Can you work these out from the drawing? Everything is in mm from the part's minimum corner. Round coordinates to 2 decimals unless told otherwise and drop trailing zeros. Write each loop counter-clockwise with the first axis right and the second up, starting at its lowest first coordinate (ties: lowest second). Pieces come first, ordered by that corner, then holes. Notation, with made-up numbers: (-18.75, 35) - (20.25, 35) arc R26 cw to (20.25, 70) - close; hole circle Ø11 at (53, 4.25). An arc over 180 degrees is marked (long way). One line per item, written item: value. Start each with the question number.
Item 1: Imagine slicing it at A-A, the plane x = 19.5. Please give me the cut outline in (y, z).
Item 2: If I drill on line 1 (Y direction, x = 19.5, z = 0.85); line 2 (X direction, y = 3.25, z = 0.35); line 3 (Z direction, x = 15.5, y = 5.5), over which ranges is the centre line in solid material (lowest first)?
Item 3: For P1, Ø1.2, axis at y = 12.5, z = 2.5, coming from the -X side; P2, Ø1.5, axis at x = 3.5, y = 19.5, coming from the -Z side; P3, Ø3, axis at x = 19.5, y = 3.5, coming from the -Z side; P4, Ø1.6, axis at y = 12, z = 2.5, coming from the +X side, each with a flat end and sliding along its axis, tell me the tip position at first contact or that it passes through.
Item 4: Imagine slicing it at C-C, the plane z = 1.2. Please give me the cut outline in (x, y), then the cut area to 3 significant figures.
Item 5: Imagine slicing it at D-D, the plane x = 10.5. Please give me the cut outline in (y, z).
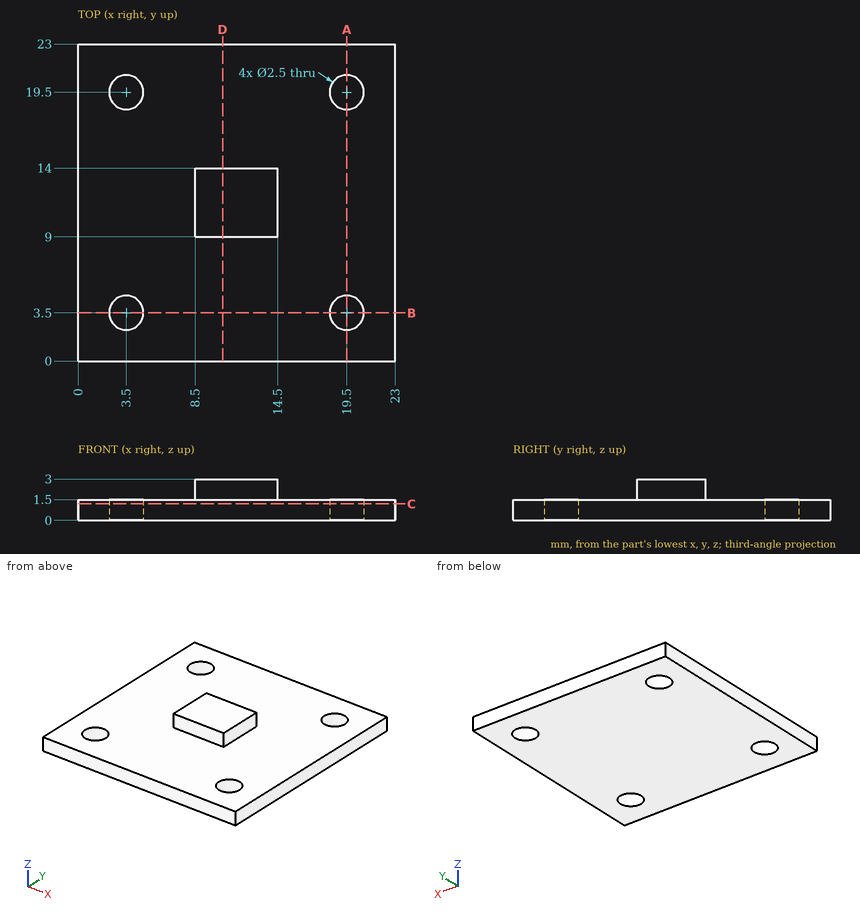
Values follow:
1. outline: (0, 0) - (2.25, 0) - (2.25, 1.5) - (0, 1.5) - close; (4.75, 0) - (18.25, 0) - (18.25, 1.5) - (4.75, 1.5) - close; (20.75, 0) - (23, 0) - (23, 1.5) - (20.75, 1.5) - close
2. line 1: y = 0 to 2.25, 4.75 to 18.25, 20.75 to 23
2. line 2: x = 0 to 2.28, 4.72 to 18.28, 20.72 to 23
2. line 3: z = 0 to 1.5
3. P1: stops at x = 8.5
3. P2: passes through
3. P3: stops at z = 0
3. P4: stops at x = 14.5
4. outline: (0, 0) - (23, 0) - (23, 23) - (0, 23) - close; hole circle Ø2.5 at (3.5, 3.5); hole circle Ø2.5 at (3.5, 19.5); hole circle Ø2.5 at (19.5, 3.5); hole circle Ø2.5 at (19.5, 19.5)
4. area: 509 mm^2
5. outline: (0, 0) - (23, 0) - (23, 1.5) - (14, 1.5) - (14, 3) - (9, 3) - (9, 1.5) - (0, 1.5) - close
